Can you work these out from the model? Positions are in its coordinate system, mm. A direction names the side the tool comes from. Round coordinates to 2 decimals unless told otherwise and drop trailing zeros. Write each loop counter-clockwise with the first axis right and the second up, starting at its lowest first coordinate (ties: lowest second). Pieces come first, ordered by that corner, then holes. Notation, with made-up numbers: (18.25, 20) -> (50.25, 20) arc R20 ccw to (50.25, 25) -> close; hole circle Ø6 at (9, -20). An arc over 180 degrees is marked (long way). Write item = value, one per line. Start each with the question number.
1) Imagine slicing it at D-D, the plane z = -86. Please give me the cut outline in (x, y), then the cut area to 3 significant figures.
2) For faces 1 (the face through (178.627, 3.219, -86.15)), 2 (the face through (53.34, 3, -249)), 3 (the face through (90, 3, -262.339)), which set-ups out of +Z, -Z, +X, -X, +Y, -Y let a thin tool reach every point of the face, with its end or its side?
3) I'm going to push a flat-ended pin straight in: pin 1 (12 mm diameter, centred on x = 122, z = -112.5, fed in from -Y). Where does the tip first touch, or does it pass through?
4) Imagine slicing it at B-B, the plane y = 1.5. State how many separate pieces and enclosed holes the cut face has, then the cut area to 3 significant figures.
5) Imagine slicing it at A-A, the plane x = 104.5. Please give me the cut outline in (y, z), then the cut area to 3 significant figures.
6) If I drill on line 1 (Z direction, x = 92, y = 4.5); line 2 (X direction, y = 4.5, z = -13.5); line 3 (Z direction, x = 22, y = 0.5), over which ranges is the centre line in solid material (lowest first)?
7) Thinking about a two-plate mould opening in X: for faces 4 (the face through (178.39, 3.22, -175.82)), 5 (the face through (93, 6.35, -133)), 6 (the face through (120.65, 3, -131)), which applies, +X half, -X half, draft (parallel to the pull), parting line (faces both ways), or undercut?
8) Imagine slicing it at C-C, the plane z = -120. Please give me the cut outline in (x, y).
from build123d import *

# Parameters (mm, degrees)
SKETCH3_R           = 1.4224
SKETCH3_W           = 6.35
SKETCH3_H           = 6.35
SKETCH3_W_2         = 76.2
SKETCH3_H_2         = 76.2
BOSS_EXTRUDE1_DEPTH = 6.35
FILLET1_R           = 10.16
FILLET2_R           = 27.94


with BuildPart() as part:
    # Sketch3 → Boss-Extrude1 (new body)
    with BuildSketch(Plane(origin=(0, 0, 0), x_dir=(1, 0, 0), z_dir=(0, 1, 0))):
        with BuildLine():
            Line((182.88, 0), (0, 0))
            Line((0, 0), (0, 262.339276313))
            Line((0, 262.339276313), (182.88, 262.339276313))
            Line((182.88, 262.339276313), (182.88, 169.269638157))
            ThreePointArc((182.88, 169.269638157), (144.78, 131.169638157), (182.88, 93.069638157))
            Line((182.88, 93.069638157), (182.88, 0))
        make_face()
        with Locations(Location((57.15, 38.1, 0), (0, 0, 270))):
            Circle(SKETCH3_R, mode=Mode.SUBTRACT)
        with Locations(Location((57.15, 114.3, 0), (0, 0, 270))):
            Circle(SKETCH3_R, mode=Mode.SUBTRACT)
        with Locations(Location((125.73, 38.1, 0), (0, 0, 90))):
            Circle(SKETCH3_R, mode=Mode.SUBTRACT)
        with Locations(Location((69.85, 151.157668748, 0), (0, 0, 270))):
            Circle(SKETCH3_R, mode=Mode.SUBTRACT)
        with Locations(Location((69.85, 219.737668748, 0), (0, 0, 270))):
            Circle(SKETCH3_R, mode=Mode.SUBTRACT)
        with Locations(Location((113.03, 151.157668748, 0), (0, 0, 90))):
            Circle(SKETCH3_R, mode=Mode.SUBTRACT)
        with Locations(Location((113.03, 219.737668748, 0), (0, 0, 90))):
            Circle(SKETCH3_R, mode=Mode.SUBTRACT)
        with Locations(Location((113.03, 42.601607565, 0), (0, 0, 270))):
            Circle(SKETCH3_R, mode=Mode.SUBTRACT)
        with Locations(Location((113.03, 111.181607565, 0), (0, 0, 270))):
            Circle(SKETCH3_R, mode=Mode.SUBTRACT)
        with Locations(Location((69.85, 111.181607565, 0), (0, 0, 90))):
            Circle(SKETCH3_R, mode=Mode.SUBTRACT)
        with Locations(Location((69.85, 42.601607565, 0), (0, 0, 90))):
            Circle(SKETCH3_R, mode=Mode.SUBTRACT)
        with Locations(Location((125.73, 224.239276313, 0), (0, 0, 270))):
            Circle(SKETCH3_R, mode=Mode.SUBTRACT)
        with Locations(Location((57.15, 224.239276313, 0), (0, 0, 90))):
            Circle(SKETCH3_R, mode=Mode.SUBTRACT)
        with Locations(Location((57.15, 148.039276313, 0), (0, 0, 90))):
            Circle(SKETCH3_R, mode=Mode.SUBTRACT)
        with Locations((22.225, 13.212735966)):
            Rectangle(SKETCH3_W, SKETCH3_H, mode=Mode.SUBTRACT)
        with Locations((160.655, 13.212735966)):
            Rectangle(SKETCH3_W, SKETCH3_H, mode=Mode.SUBTRACT)
        with Locations((160.655, 249.126540348)):
            Rectangle(SKETCH3_W, SKETCH3_H, mode=Mode.SUBTRACT)
        with Locations((22.225, 249.126540348)):
            Rectangle(SKETCH3_W, SKETCH3_H, mode=Mode.SUBTRACT)
        with Locations((91.44, 249.126540348)):
            Rectangle(SKETCH3_W_2, SKETCH3_H, mode=Mode.SUBTRACT)
        with Locations((91.44, 13.212735966)):
            Rectangle(SKETCH3_W_2, SKETCH3_H, mode=Mode.SUBTRACT)
        with Locations((123.825, 131.169638157)):
            Rectangle(SKETCH3_W, SKETCH3_H_2, mode=Mode.SUBTRACT)
        with Locations((22.225, 131.169638157)):
            Rectangle(SKETCH3_W, SKETCH3_H_2, mode=Mode.SUBTRACT)
    extrude(amount=BOSS_EXTRUDE1_DEPTH)

    # Fillet1
    fillet1_edges = [part.edges().sort_by_distance(p)[0] for p in [
        (0, 3.175, -262.339276313),
        (182.88, 3.175, -262.339276313),
        (182.88, 3.175, 0),
        (0, 3.175, 0),
    ]]
    fillet(fillet1_edges, radius=FILLET1_R)

    # Fillet2
    fillet2_edges = [part.edges().sort_by_distance(p)[0] for p in [
        (182.88, 3.175, -169.269638157),
        (182.88, 3.175, -93.069638157),
    ]]
    fillet(fillet2_edges, radius=FILLET2_R)


solid = part.part
Reported:
q1.outline = (0, 0) -> (178.72, 0) -> (178.72, 6.35) -> (0, 6.35) -> close
q1.area = 1,130 mm²
q2.face_1 = +X, +Y, -Y
q2.face_2 = +Y, -Y
q2.face_3 = -Z, +X, -X, +Y, -Y
q3.pin_1 = 0
q4.separate_pieces = 1
q4.enclosed_holes = 22
q4.area = 43,300 mm²
q5.outline = (0, -262.34) -> (6.35, -262.34) -> (6.35, -252.3) -> (0, -252.3) -> close; (0, -245.95) -> (6.35, -245.95) -> (6.35, -16.39) -> (0, -16.39) -> close; (0, -10.04) -> (6.35, -10.04) -> (6.35, 0) -> (0, 0) -> close
q5.area = 1,590 mm²
q6.line_1 = -262.34 to -252.3, -245.95 to -16.39, -10.04 to 0
q6.line_2 = 0 to 19.05, 25.4 to 53.34, 129.54 to 157.48, 163.83 to 182.88
q6.line_3 = -262.34 to -252.3, -245.95 to -169.27, -93.07 to -16.39, -10.04 to 0
q7.face_4 = +X half
q7.face_5 = draft
q7.face_6 = undercut
q8.outline = (0, 0) -> (19.05, 0) -> (19.05, 6.35) -> (0, 6.35) -> close; (25.4, 0) -> (120.65, 0) -> (120.65, 6.35) -> (25.4, 6.35) -> close; (127, 0) -> (146.45, 0) -> (146.45, 6.35) -> (127, 6.35) -> close
